Can you work these out from the model? Positions are in its coordinate system, mm. Face numbers are marked on the shaded views. Give positions to 0.01 mm unless a question says otherwise; leave off trailing zeros. Order: outer loops, then holes, each group sorted by start corner. A loop starts at its lowest first (then second) coordinate and runs counter-clockwise, first axis right, second up. Notation, with made-up numbers: M 0.5,-16 L 31.5,-16 A23 cw 31.5,-6 Z; hole C 76,-2 d7. An arc over 180 degrees is marked long. Use one line per item in the form item = value. Start each with the question number.
1. We'd pull the mould along X, two halves only. Please class the marked faces 1 and 2: +X half, -X half, draft (parallel to the pull), parting line (faces both ways), or undercut.
2. I want a section at D-D, the plane z = 0.9. List the corners of the cut face in (x, y) for me, and give its area (3 significant figures).
3. I want a section at C-C, the plane z = 0.25. List the corners of the cut face in (x, y) for me, and give its area (3 significant figures).
4. I need wall thicknesses on L1, parallel to Y at x = 0, z = 0.5; L2, parallel to X at y = -1, z = 0.95; L3, parallel to Z at x = -5, y = -3.5. Which ranges of each line are inside material? Lowest first, please.
5. I want a section at A-A, the plane y = 0. List the corners of the cut face in (x, z) for me (3 decimals), and give its area (3 significant figures).
6. Will these pins go through, and if not, where does the flat tip stop? P1, Ø1.5, axis at x = -1.5, z = 1, coming from the -Y side; P2, Ø1.5, axis at y = 3, z = 2, coming from the -X side.
```python
from build123d import *

# Parameters (mm, degrees)
F0_R     = 6.35
F1_DEPTH = 2.54
F2_R     = 0.635
F4_R     = 1.27
F5_DEPTH = 2.54


with BuildPart() as f1:
    # F0 (on Top) → F1 (new body)
    with BuildSketch(Plane.XY):
        Circle(F0_R)
    extrude(amount=F1_DEPTH)

    # F2 (on Front) → F3 (revolve, cut)
    with BuildSketch(Plane.XZ):
        with Locations((-6.370238, 1.27)):
            Circle(F2_R)
    revolve(axis=Axis((0, 0, 2.54), (0, 0, 1)), mode=Mode.SUBTRACT)

    # F4 (on face) → F5 (cut)
    with BuildSketch(Plane.XY.offset(2.54)):
        Circle(F4_R)
    extrude(amount=-F5_DEPTH, mode=Mode.SUBTRACT)


solid = f1.part
```
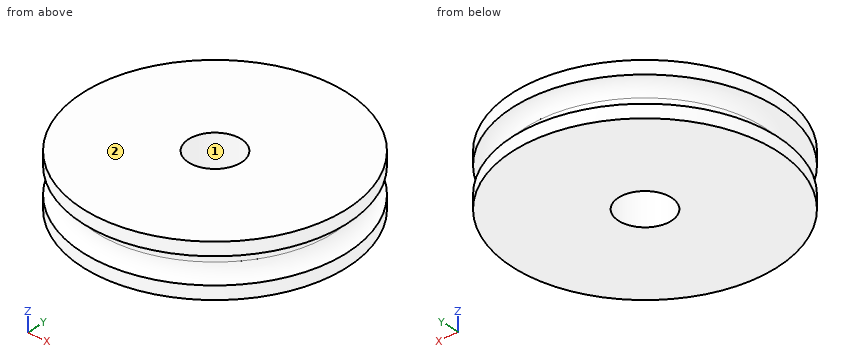
Check result:
q1.face_1 = undercut
q1.face_2 = draft
q2.outline = C 0,0 d11.71; hole C 0,0 d2.54
q2.area = 103 mm2
q3.outline = C 0,0 d12.7; hole C 0,0 d2.54
q3.area = 122 mm2
q4.L1 = -6.35 to -1.27, 1.27 to 6.35
q4.L2 = -5.74 to -0.78, 0.78 to 5.74
q4.L3 = 0 to 0.69, 1.85 to 2.54
q5.outline = M -6.35,0 L -1.27,0 L -1.27,2.54 L -6.35,2.54 L -6.35,1.905 A0.635 cw -6.35,0.635 Z; M 1.27,0 L 6.35,0 L 6.35,0.635 A0.635 cw 6.35,1.905 L 6.35,2.54 L 1.27,2.54 Z
q5.area = 24.6 mm2
q6.P1 = -6.29
q6.P2 = -5.94
